The listing builds one solid part. Answer for the finished solid, in the listing's coordinates (mm). A direction names the side the tool comes from. Round coordinates to 2 decimals unless told otherwise and drop trailing zeros. Write each loop counter-clockwise with the first axis right and the second up, starting at its lowest first coordinate (ties: lowest second). Pieces come first, ordered by that corner, then holes. Notation, with made-up numbers: M -2.75,-38.75 L 40.25,-38.75 A23 cw 40.25,-12.75 Z; hole C -0.5,-18 d3. An arc over 180 degrees is marked long. Write each question's results on one line, items separated by ' | '.
from build123d import *

# Parameters (mm, degrees)
SKETCH1_W               = 30
SKETCH1_H               = 30
SKETCH1_W_2             = 26
SKETCH1_H_2             = 26
BOSS_EXTRUDE1_DEPTH     = 550
CUT_EXTRUDE1_DEPTH      = 552.633936592
CUT_EXTRUDE1_DEPTH_BACK = 552.633936592
SKETCH2_R               = 4


with BuildPart() as part:
    # Sketch1 → Boss-Extrude1 (new body)
    with BuildSketch(Plane(origin=(0, 0, 0), x_dir=(0, 0, -1), z_dir=(1, 0, 0))):
        with Locations((15, 15)):
            Rectangle(SKETCH1_W, SKETCH1_H)
        with Locations((15, 15)):
            Rectangle(SKETCH1_W_2, SKETCH1_H_2, mode=Mode.SUBTRACT)
    extrude(amount=BOSS_EXTRUDE1_DEPTH)

    # Sketch2 → Cut-Extrude1 (cut, two sides: drawn at the far end of the back side and taken through both)
    with BuildSketch(Plane.XY.offset(-CUT_EXTRUDE1_DEPTH_BACK)):
        with Locations((15, 15)):
            Circle(SKETCH2_R)
        with Locations((440, 15)):
            Circle(SKETCH2_R)
        with Locations((540, 15)):
            Circle(SKETCH2_R)
    extrude(amount=CUT_EXTRUDE1_DEPTH + CUT_EXTRUDE1_DEPTH_BACK, mode=Mode.SUBTRACT)


solid = part.part
1) A tool of negligible diameter and unlimited length cuts with its end or side. For faces 1 (the face through (271, 2, -15)), 2 (the face through (0, 15, -1)), from which of +Z, -Z, +X, -X, +Y, -Y can it reach the whole face along a straight path? Write none if from no direction.
Return value:
face 1: +X, -X | face 2: +Z, -Z, -X, +Y, -Y
2) Section A-A (z = -20.5) is taken. Determine the outline of the cut face in (x, y), then the cut area to 3 significant figures.
Return value:
outline: M 0,0 L 550,0 L 550,2 L 0,2 Z; M 0,28 L 550,28 L 550,30 L 0,30 Z | area: 2,200 mm²
3) Find the intervals of material crossed by line 1 (X direction, y = 15, z = -29.35); line 2 (Y direction, x = 431, z = -6.75); line 3 (Z direction, x = 105, y = 27), in increasing order.
Return value:
line 1: 0 to 11, 19 to 436, 444 to 536, 544 to 550 | line 2: 0 to 2, 28 to 30 | line 3: -30 to -28, -2 to 0
4) This flat-tipped pin is pushed along its axis until it touches: pin 1 (6.5 mm diameter, centred on x = 440, y = 15, fed in from +Z). Where does it stop, or does it pass through?
Return value:
pin 1: through
5) The mould has two halves that part along Z. Classify faces 3 (the face through (271, 0, -15)), 4 (the face through (271, 15, -30)), 5 (the face through (271, 15, 0)), 6 (the face through (271, 15, -28)): +Z half, -Z half, draft (parallel to the pull), parting line (faces both ways), or undercut.
Return value:
face 3: draft | face 4: -Z half | face 5: +Z half | face 6: undercut
6) Section B-B (x = 264) is taken. Determine the outline of the cut face in (y, z).
Return value:
outline: M 0,-30 L 30,-30 L 30,0 L 0,0 Z; hole M 2,-28 L 28,-28 L 28,-2 L 2,-2 Z
